Geometry: final body of the model. Coordinates: model frame, mm. Coordinates: 2 decimals unless noted, no trailing zeros. Order: outer loops, then holes, each group sorted by start corner. A loop starts at its lowest first (then second) coordinate and runs counter-clockwise, first axis right, second up. Notation, with made-up numbers: (-16.5, 16.5) -> (10.5, 16.5) arc R25 ccw to (10.5, 43.5) -> close; hole circle Ø1 at (17.5, 28). An arc over 180 degrees is marked (long way). Use one line per item in the form item = value.
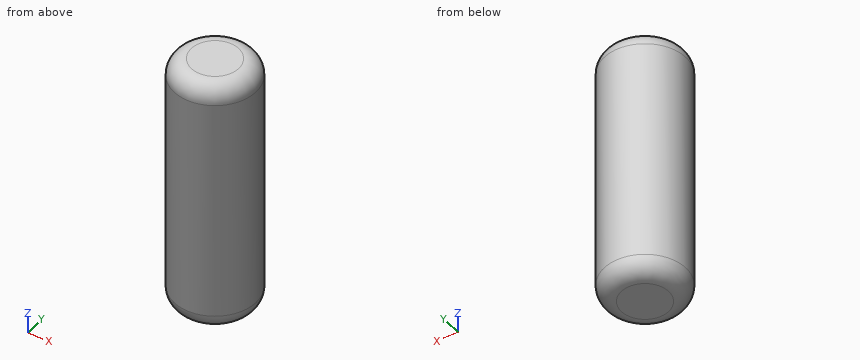
```python
from build123d import *

# Parameters (mm, degrees)
SKETCH1_R           = 120.65
BOSS_EXTRUDE1_DEPTH = 762
FILLET2_R           = 50.8
CUT_EXTRUDE1_START  = -25.4
SKETCH2_R           = 101.6
CUT_EXTRUDE1_DEPTH  = 711.2


with BuildPart() as part:
    # Sketch1 → Boss-Extrude1 (new body)
    with BuildSketch(Plane.XY):
        Circle(SKETCH1_R)
    extrude(amount=BOSS_EXTRUDE1_DEPTH)

    # Fillet2
    fillet2_edges = [part.edges().sort_by_distance(p)[0] for p in [
        (-120.65, 0, 0),
        (-120.65, 0, 762),
    ]]
    fillet(fillet2_edges, radius=FILLET2_R)

    # Sketch2 → Cut-Extrude1 (cut)
    with BuildSketch(Plane.XY.offset(762).offset(CUT_EXTRUDE1_START)):
        Circle(SKETCH2_R)
    extrude(amount=-CUT_EXTRUDE1_DEPTH, mode=Mode.SUBTRACT)


solid = part.part
```
1) Section A-A, the plane x = 0. Output: boundary loops of the cut face in (y, z), and give its area (3 significant figures).
Results found:
outline = (-120.65, 50.8) arc R50.8 ccw to (-69.85, 0) -> (69.85, 0) arc R50.8 ccw to (120.65, 50.8) -> (120.65, 711.2) arc R50.8 ccw to (69.85, 762) -> (-69.85, 762) arc R50.8 ccw to (-120.65, 711.2) -> close; hole (-101.6, 25.4) -> (101.6, 25.4) -> (101.6, 736.6) -> (-101.6, 736.6) -> close
area = 37,100 mm2
2) Section C-C, the plane z = 156. Output: boundary loops of the cut face in (x, y).
Results found:
outline = circle Ø241.3 at (0, 0); hole circle Ø203.2 at (0, 0)
3) Material intervals for probe 1 along Z at (x, y) = (10.5, -26.5); probe 2 along Y at (x, z) = (0, 335.5); probe 3 along X at (y, z) = (65, 248), sorted ascending. Write a range as from..to.
Results found:
probe_1 = 0..25.4, 736.6..762
probe_2 = -120.65..-101.6, 101.6..120.65
probe_3 = -101.64..-78.09, 78.09..101.64
4) Contact query for flat-ended pins moving along their axis: P1, Ø3, axis at x = -31.5, z = 605, coming from the -Y side; P2, Ø3, axis at x = 79, y = -86.5, coming from the +Z side (3 decimals); P3, Ø10, axis at y = 55.5, z = 627, coming from the +X side. Output: stop coordinate, or through.
Results found:
P1 = -116.86
P2 = 733.185
P3 = 109.57
